Here's how the part is built. I have some questions about the finished solid (model axes, mm). A direction names the side the tool comes from. Give positions to 0.01 mm unless a question says otherwise; leave off trailing zeros. Order: outer loops, then holes, each group sorted by start corner. A loop starts at its lowest first (then second) coordinate and runs counter-clockwise, first axis right, second up. Notation, with made-up numbers: (60.25, -19) -> (80.25, -19) arc R32 cw to (80.25, 18) -> close; hole circle Ø9 at (57, 69). An arc over 180 degrees is marked (long way). Write each question's results on one line, items separated by ' | '. Start each with the question number.
Q1. Thinking about a two-plate mould opening in X: for faces 1 (the face through (85.75, 24.35, 12.98)), 2 (the face through (93, 13, 6)), 3 (the face through (-33.221, 24.886, 12.979)), 4 (the face through (-20, 2, 0)), which applies, pulls with the +X half, pulls with the -X half, needs draft (parallel to the pull), parting line crosses it, or undercut?
Q2. Imagine slicing it at B-B, the plane x = 59. Please give me the cut outline in (y, z).
Q3. For faces 5 (the face through (25, 2, 5)), 6 (the face through (54, 2, 19)), 7 (the face through (87, 14, 7.5)), 8 (the face through (-27, 12, 13)), which set-ups out of +Z, -Z, +X, -X, +Y, -Y let a thin tool reach every point of the face, with its end or its side?
Q4. I need wall thicknesses on line 1 along X through (y, z) = (5.5, 6.3); line 2 along X through (y, z) = (14.5, 7); line 3 along X through (y, z) = (23.2, 12.65). Which ranges of each line are inside material? Lowest first, please. Write a range as [from, to].
Q5. Imagine slicing it at A-A, the plane z = 9.25. Please give me the cut outline in (x, y).
Q6. Imagine slicing it at C-C, the plane y = 16.5. Please give me the cut outline in (x, z), then the cut area to 3 significant figures.
Q7. Imagine slicing it at D-D, the plane z = 16.25. Please give me the cut outline in (x, y), then the cut area to 3 significant figures.
Q8. I'm going to push flat-ended pins straight in: pin 1 (4 mm diameter, centred on x = -18, z = 19, fed in from -Y); pin 2 (0.9 mm diameter, centred on y = 8.5, z = -1.5, fed in from -X); pin 3 (9.5 mm diameter, centred on x = 87.5, y = 13.5, fed in from +Z); pin 4 (1.5 mm diameter, centred on x = 85, z = 12.5, fed in from +Y). Where does each tip first touch, or does it pass through?
```python
from build123d import *

# Parameters (mm, degrees)
BOX009_W          = 95
BOX009_H          = 5
BOX009_DEPTH      = 9
CYLINDER001_R     = 1.7
CYLINDER001_DEPTH = 31
CYLINDER_R        = 1.7
CYLINDER_DEPTH    = 31
BOX005_W          = 12
BOX005_H          = 27
BOX005_DEPTH      = 3
BOX006_W          = 12
BOX006_H          = 27
BOX006_DEPTH      = 3
BOX007_W          = 12
BOX007_H          = 27
BOX007_DEPTH      = 3
BOX003_W          = 3
BOX003_H          = 30
BOX003_DEPTH      = 19
BOX001_W          = 12
BOX001_H          = 27
BOX001_DEPTH      = 3
BOX002_W          = 12
BOX002_H          = 27
BOX002_DEPTH      = 3
BOX008_W          = 12
BOX008_H          = 10
BOX008_DEPTH      = 4
BOX_W             = 117
BOX_H             = 3
BOX_DEPTH         = 19
BOX004_W          = 12
BOX004_H          = 27
BOX004_DEPTH      = 3
FILLET_R          = 5


with BuildPart() as cube009:
    # Box009 → Box009 (new body)
    with BuildSketch(Plane(origin=(-22, 0, 5), x_dir=(1, 0, 0), z_dir=(0, 0, 1))):
        with Locations((47.5, 2.5)):
            Rectangle(BOX009_W, BOX009_H)
    extrude(amount=BOX009_DEPTH)


with BuildPart() as cylinder001:
    # Cylinder001 → Cylinder001 (new body)
    with BuildSketch(Plane(origin=(6, 23.2, -6), x_dir=(1, 0, 0), z_dir=(0, 0, 1))):
        Circle(CYLINDER001_R)
    extrude(amount=CYLINDER001_DEPTH)


with BuildPart() as cylinder:
    # Cylinder → Cylinder (new body)
    with BuildSketch(Plane(origin=(6, 5.5, -6), x_dir=(1, 0, 0), z_dir=(0, 0, 1))):
        Circle(CYLINDER_R)
    extrude(amount=CYLINDER_DEPTH)


with BuildPart() as fusion002:
    # Fusion002 base: copy of Cylinder
    add(cylinder.part)

    # Fusion002: union Cylinder001
    add(cylinder001.part)


with BuildPart() as fusion002_1:
    # Fusion002 placement: moved
    add(fusion002.part.moved(Location((81, 0, 0))))


with BuildPart() as fusion003:
    # Fusion003 base: copy of Cylinder
    add(cylinder.part)

    # Fusion003: union Cylinder001
    add(cylinder001.part)


with BuildPart() as fusion003_1:
    # Fusion003 placement: moved
    add(fusion003.part.moved(Location((-39, 0, 0))))


with BuildPart() as obj1:
    # Fusion001 base: copy of Cylinder
    add(cylinder.part)

    # Fusion001: union Cylinder001
    add(cylinder001.part)

    # Fusion004: union Fusion002, Fusion003
    add(fusion002_1.part)
    add(fusion003_1.part)


with BuildPart() as cube005:
    # Box005 → Box005 (new body)
    with BuildSketch(Plane(origin=(-39, 0, 11.5), x_dir=(1, 0, 0), z_dir=(0, 0, 1))):
        with Locations((6, 13.5)):
            Rectangle(BOX005_W, BOX005_H)
    extrude(amount=BOX005_DEPTH)


with BuildPart() as cube006:
    # Box006 → Box006 (new body)
    with BuildSketch(Plane(origin=(81, 0, 4.5), x_dir=(1, 0, 0), z_dir=(0, 0, 1))):
        with Locations((6, 13.5)):
            Rectangle(BOX006_W, BOX006_H)
    extrude(amount=BOX006_DEPTH)


with BuildPart() as cube007:
    # Box007 → Box007 (new body)
    with BuildSketch(Plane(origin=(81, 0, 11.5), x_dir=(1, 0, 0), z_dir=(0, 0, 1))):
        with Locations((6, 13.5)):
            Rectangle(BOX007_W, BOX007_H)
    extrude(amount=BOX007_DEPTH)


with BuildPart() as cube003:
    # Box003 → Box003 (new body)
    with BuildSketch(Plane(origin=(78, 0, 0), x_dir=(1, 0, 0), z_dir=(0, 0, 1))):
        with Locations((1.5, 15)):
            Rectangle(BOX003_W, BOX003_H)
    extrude(amount=BOX003_DEPTH)


with BuildPart() as cube001:
    # Box001 → Box001 (new body)
    with BuildSketch(Plane.XY.offset(-3)):
        with Locations((6, 13.5)):
            Rectangle(BOX001_W, BOX001_H)
    extrude(amount=BOX001_DEPTH)


with BuildPart() as cube002:
    # Box002 → Box002 (new body)
    with BuildSketch(Plane.XY.offset(19)):
        with Locations((6, 13.5)):
            Rectangle(BOX002_W, BOX002_H)
    extrude(amount=BOX002_DEPTH)


with BuildPart() as cube008:
    # Box008 → Box008 (new body)
    with BuildSketch(Plane(origin=(-39, -7, 7.5), x_dir=(1, 0, 0), z_dir=(0, 0, 1))):
        with Locations((6, 5)):
            Rectangle(BOX008_W, BOX008_H)
    extrude(amount=BOX008_DEPTH)


with BuildPart() as cut:
    # Box → Box (new body)
    with BuildSketch(Plane(origin=(-39, 0, 0), x_dir=(1, 0, 0), z_dir=(0, 0, 1))):
        with Locations((58.5, 1.5)):
            Rectangle(BOX_W, BOX_H)
    extrude(amount=BOX_DEPTH)

    # Cut: cut Cube008
    add(cube008.part, mode=Mode.SUBTRACT)


with BuildPart() as cut002:
    # Box004 → Box004 (new body)
    with BuildSketch(Plane(origin=(-39, 0, 4.5), x_dir=(1, 0, 0), z_dir=(0, 0, 1))):
        with Locations((6, 13.5)):
            Rectangle(BOX004_W, BOX004_H)
    extrude(amount=BOX004_DEPTH)

    # Fusion: union Cube005, Cube006, Cube007, Cube003, Cube001, Cube002, Cut
    add(cube005.part)
    add(cube006.part)
    add(cube007.part)
    add(cube003.part)
    add(cube001.part)
    add(cube002.part)
    add(cut.part)

    # Cut001: cut obj1
    add(obj1.part, mode=Mode.SUBTRACT)

    # Fillet
    fillet_edges = [cut002.edges().sort_by_distance(p)[0] for p in [
        (93, 0, 6),
        (93, 0, 13),
        (93, 27, 6),
        (93, 27, 13),
        (79.5, 30, 19),
        (79.5, 30, 0),
        (0, 27, 20.5),
        (-39, 27, 13),
        (-39, 27, 6),
        (0, 27, -1.5),
        (12, 27, -1.5),
        (12, 27, 20.5),
        (-27, 27, 13),
        (-27, 27, 6),
    ]]
    fillet(fillet_edges, radius=FILLET_R)

    # Cut002: cut Cube009
    add(cube009.part, mode=Mode.SUBTRACT)


solid = cut002.part
```
Geometry check:
1) face 1: undercut | face 2: pulls with the +X half | face 3: undercut | face 4: needs draft
2) outline: (0, 0) -> (3, 0) -> (3, 5) -> (0, 5) -> close; (0, 14) -> (3, 14) -> (3, 19) -> (0, 19) -> close
3) face 5: +Y, -Y | face 6: +Z, +X, +Y, -Y | face 7: +X, +Y, -Y | face 8: +Z, -Z, +Y
4) line 1: [-39, -34.7], [-31.3, -27], [78, 85.3], [88.7, 93] | line 2: [-39, -27], [78, 93] | line 3: [-38.85, -34.7], [-31.3, -27.15], [78, 85.3], [88.7, 92.85]
5) outline: (-27, 0) -> (-22, 0) -> (-22, 3) -> (-27, 3) -> close; (73, 0) -> (81, 0) -> (81, 30) -> (78, 30) -> (78, 3) -> (73, 3) -> close
6) outline: (-39, 4.5) -> (-27, 4.5) -> (-27, 7.5) -> (-39, 7.5) -> close; (-39, 11.5) -> (-27, 11.5) -> (-27, 14.5) -> (-39, 14.5) -> close; (0, -3) -> (12, -3) -> (12, 0) -> (0, 0) -> close; (0, 19) -> (12, 19) -> (12, 22) -> (0, 22) -> close; (78, 0) -> (81, 0) -> (81, 4.5) -> (93, 4.5) -> (93, 7.5) -> (81, 7.5) -> (81, 11.5) -> (93, 11.5) -> (93, 14.5) -> (81, 14.5) -> (81, 19) -> (78, 19) -> close | area: 273 mm²
7) outline: (-39, 0) -> (81, 0) -> (81, 29.47) -> (78, 29.47) -> (78, 3) -> (-39, 3) -> close | area: 439 mm²
8) pin 1: y = 0 | pin 2: x = 0 | pin 3: z = 14.5 | pin 4: y = 27
